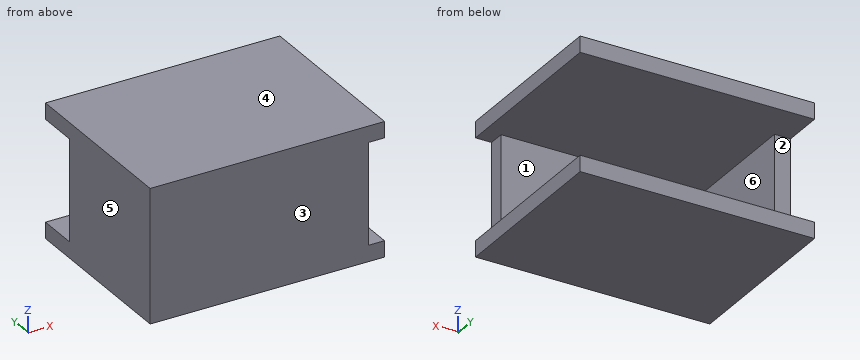
Autodesk Inventor part; units mm, degrees
ref_plane "YZ Plane" through (0, 0, 0) normal (1, 0, 0) x (0, 1, 0)
ref_plane "XZ Plane" through (0, 0, 0) normal (0, 1, 0) x (-1, 0, 0)
ref_plane "XY Plane" through (0, 0, 0) normal (0, 0, 1) x (1, 0, 0)
sketch "Sketch2" plane through (0, 0, 0) normal (0, 1, 0) x (-1, 0, 0)
  line L0 (0, 0) -> (40, 0)
  line L1 (40, 0) -> (40, -20)
  line L2 (40, -20) -> (0, -20)
  line L3 (0, -20) -> (0, 0)
  dimension "d25" = 40
  dimension "d26" = 20
extrude "Extrusion1" add sketch "Sketch2" along normal blind 3.18
sketch "Sketch5" plane through (0, 0, 0) normal (0, 1, 0) x (-1, 0, 0)
  line L0 (40, 0) -> (0, 0)
  line L1 (0, 0) -> (0, -20)
  line L2 (0, -20) -> (40, -20)
  line L3 (40, -20) -> (40, 0)
  line L4 (-3.18, 0) -> (43.18, 0)
  line L5 (43.18, 0) -> (43.18, 3.18)
  line L6 (43.18, 3.18) -> (-3.18, 3.18)
  line L7 (-3.18, 3.18) -> (-3.18, 0)
  line L8 (43.18, -20) -> (-3.18, -20)
  line L9 (-3.18, -20) -> (-3.18, -23.18)
  line L10 (-3.18, -23.18) -> (43.18, -23.18)
  line L11 (43.18, -23.18) -> (43.18, -20)
  dimension "d34" = 3.18
  dimension "d35" = 3.18
  dimension "d36" = 3.18
extrude "Extrusion2" add sketch "Sketch5" along normal blind 35 contours L0 L4 L7 L6 L5 | L8 L11 L10 L9 L2
sketch "Sketch6" plane through (0, 0, 0) normal (0, 1, 0) x (-1, 0, 0)
  line L0 (40, 0) -> (0, 0)
  line L1 (0, 0) -> (0, -20)
  line L2 (0, -20) -> (40, -20)
  line L3 (40, -20) -> (40, 0)
  line L4 (40, 0) -> (43.18, 0)
  line L5 (43.18, 0) -> (43.18, -20)
  line L6 (43.18, -20) -> (40, -20)
  line L7 (40, -20) -> (40, 0)
  dimension "d39" = 3.18
  dimension "d40" = 20
extrude "Extrusion3" add sketch "Sketch6" along normal blind 27 contours L4 L5 L6 L3
properties part number "Base_servo1"
Part model, mm, in its own coordinate system. Face numbers are marked on the shaded views. A direction names the side the tool comes from. Round coordinates to 2 decimals unless told otherwise and drop trailing zeros. Order: outer loops, then holes, each group sorted by start corner. A loop starts at its lowest first (then second) coordinate and runs counter-clockwise, first axis right, second up. Notation, with made-up numbers: M -14.75,80.25 L 31.25,80.25 A22 cw 31.25,93.25 Z; hole C 77.5,25.5 d5. An arc over 180 degrees is marked long. Put each result on its own line as item: value. Start each with the question number.
1. Slice it at D-D on x = -36. List the corners of the cut face in (y, z).
2. Two-plate mould, pull along Z, no slides. Class the marked faces 4, 5 and 6: +Z half, -Z half, draft (parallel to the pull), parting line (faces both ways), or undercut.
3. Slice it at C-C on z = -5.5. List the corners of the cut face in (x, y).
4. Tool access for the marked faces 1, 2 and 3: list every direction of +Z, -Z, +X, -X, +Y, -Y with a clear straight run to the whole face (end or side of a thin tool).
5. Slice it at A-A on y = 28.5. List the corners of the cut face in (x, z), then the cut area to 3 significant figures.
6. Slice it at B-B on y = 24.5. List the corners of the cut face in (x, z).
7. Drill centre lines: probe 1 along Z at (x, y) = (-36, 18); probe 2 along X at (y, z) = (20, -6); probe 3 along Y at (x, z) = (-18.5, -18.75). Where is each one in solid material? Low to high. Write a range as [from, to].
8. Drop flat-ended pins along their axis: pin 1 (6 mm diameter, centred on y = 19, z = -7, fed in from +X); pin 2 (2.5 mm diameter, centred on y = 1.5, z = -6, fed in from +X); pin 3 (1.6 mm diameter, centred on x = -42, z = -15, fed in from +Y). Give the stop position or say it passes through.
Findings:
1. outline: M 0,-23.18 L 35,-23.18 L 35,-20 L 3.18,-20 L 3.18,0 L 35,0 L 35,3.18 L 0,3.18 Z
2. face 4: +Z half
2. face 5: draft
2. face 6: undercut
3. outline: M -43.18,0 L 0,0 L 0,3.18 L -40,3.18 L -40,27 L -43.18,27 Z
4. face 1: +X, +Y
4. face 2: +X, -X, +Y
4. face 3: +Z, -Z, +X, -X, -Y
5. outline: M -43.18,-23.18 L 3.18,-23.18 L 3.18,-20 L -43.18,-20 Z; M -43.18,0 L 3.18,0 L 3.18,3.18 L -43.18,3.18 Z
5. area: 295 mm2
6. outline: M -43.18,-23.18 L 3.18,-23.18 L 3.18,-20 L -40,-20 L -40,0 L 3.18,0 L 3.18,3.18 L -43.18,3.18 Z
7. probe 1: [-23.18, -20], [0, 3.18]
7. probe 2: [-43.18, -40]
7. probe 3: [0, 3.18]
8. pin 1: x = -40
8. pin 2: x = 0
8. pin 3: y = 27
